Input: part model. Units: mm. Frame: model coordinates. Face numbers are marked on the shaded views. A direction names the side the tool comes from. Give positions to 0.01 mm unless a question says otherwise; leave off trailing zeros. Loops run counter-clockwise (first coordinate to the right, second up) from the corner with the lowest first, then second, coordinate; pieces in that order, holes last.
from build123d import *

# Parameters (mm, degrees)
SKETCH1_R           = 1.65
BOSS_EXTRUDE1_DEPTH = 16
SKETCH2_R           = 2.55
BOSS_EXTRUDE2_DEPTH = 1.5
FILLET1_R           = 2


with BuildPart() as part:
    # Sketch1 → Boss-Extrude1 (new body)
    with BuildSketch(Plane(origin=(76, 0, 0), x_dir=(0, 0, -1), z_dir=(1, 0, 0))):
        Polygon((-39.367141304, -29.396728555), (-62.367141304, -29.396728555), (-62.367141304, -3.396728555), (-56.367141304, -3.396728555), (-56.367141304, -19.796728555), (-39.367141304, -19.796728555), align=None)
        with Locations(Location((-59.367141305, -24.59672823, 0), (0, 0, 90))):
            Circle(SKETCH1_R, mode=Mode.SUBTRACT)
        with Locations(Location((-59.367141305, -6.59672823, 0), (0, 0, 90))):
            Circle(SKETCH1_R, mode=Mode.SUBTRACT)
    extrude(amount=-BOSS_EXTRUDE1_DEPTH)

    # Sketch2 → Boss-Extrude2 (add)
    with BuildSketch(Plane(origin=(0, -19.796728555, 0), x_dir=(1, 0, 0), z_dir=(0, 1, 0))):
        with Locations(Location((64, -51.367141304, 0), (0, 0, 270))):
            Circle(SKETCH2_R)
        with Locations(Location((64, -43.367141304, 0), (0, 0, 270))):
            Circle(SKETCH2_R)
        with Locations(Location((72, -43.367141304, 0), (0, 0, 270))):
            Circle(SKETCH2_R)
        with Locations(Location((72, -51.367141304, 0), (0, 0, 270))):
            Circle(SKETCH2_R)
    extrude(amount=BOSS_EXTRUDE2_DEPTH)

    # Fillet1
    fillet1_edges = [part.edges().sort_by_distance(p)[0] for p in [
        (68, -29.396728555, 62.367141304),
        (68, -3.396728555, 62.367141304),
        (68, -3.396728555, 56.367141304),
    ]]
    fillet(fillet1_edges, radius=FILLET1_R)


solid = part.part
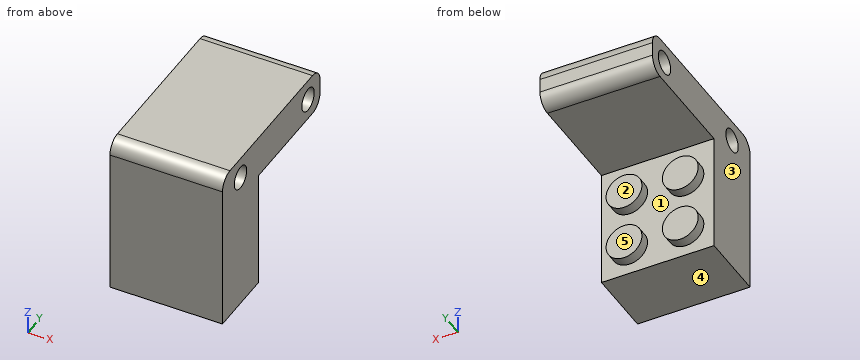
(1) Cut plane A-A (y = -23.75). Return the cut outline in (x, z).
Values follow:
outline: (60, 39.37) - (76, 39.37) - (76, 57.95) - (60, 57.95) - close; (60, 60.78) - (76, 60.78) - (76, 62.37) - (60, 62.37) - close
(2) Ray query, probe 1 along Y at (x, z) = (71.75, 49.75); probe 2 along Z at (x, y) = (66.25, -19.5); probe 3 along Y at (x, z) = (63, 47.75). Return the intervals inside material, ascending.
Values follow:
probe 1: y = -29.4 to -18.3
probe 2: z = 42.17 to 44.57, 50.17 to 52.57, 56.37 to 62.37
probe 3: y = -29.4 to -19.8
(3) Cut plane B-B (x = 72). Return the cut outline in (y, z).
Values follow:
outline: (-29.4, 39.37) - (-19.8, 39.37) - (-19.8, 40.82) - (-18.3, 40.82) - (-18.3, 45.92) - (-19.8, 45.92) - (-19.8, 48.82) - (-18.3, 48.82) - (-18.3, 53.92) - (-19.8, 53.92) - (-19.8, 56.37) - (-5.4, 56.37) arc R2 ccw to (-3.4, 58.37) - (-3.4, 60.37) arc R2 ccw to (-5.4, 62.37) - (-27.4, 62.37) arc R2 ccw to (-29.4, 60.37) - close; hole circle Ø3.3 at (-24.6, 59.37); hole circle Ø3.3 at (-6.6, 59.37)
(4) Cut plane C-C (z = 43.25). Return the cut outline in (x, y).
Values follow:
outline: (60, -29.4) - (76, -29.4) - (76, -19.8) - (74.55, -19.8) - (74.55, -18.3) - (69.45, -18.3) - (69.45, -19.8) - (66.55, -19.8) - (66.55, -18.3) - (61.45, -18.3) - (61.45, -19.8) - (60, -19.8) - close
(5) Reachability of the marked faces 4 and 5 from +Z, -Z, +X, -X, +Y, -Y: full face, straight path, thin tool, end or side. Return the list, or none.
Values follow:
face 4: -Z, +X, -X, +Y, -Y
face 5: -Z, +X, -X, +Y
(6) Cut plane D-D (y = -11.5). Return the cut outline in (x, z).
Values follow:
outline: (60, 56.37) - (76, 56.37) - (76, 62.37) - (60, 62.37) - close
(7) Pin query (flat end, axial travel): pin 1 Ø4 at (x, z) = (73, 42) entering from +Y; pin 2 Ø1 at (x, y) = (65.5, -10.5) entering from -Z; pin 3 Ø1.5 at (x, z) = (73.5, 57) entering from +Y. Return the tip coordinate at first contact, or that it passes through.
Values follow:
pin 1: stops at y = -18.3
pin 2: stops at z = 56.37
pin 3: stops at y = -3.49
(8) Mould query, pull axis X, two halves, no side actions, for the marked faces 1, 2 and 3. Classes: +X half, -X half, draft (parallel to the pull), parting line (faces both ways), or undercut.
Values follow:
face 1: undercut
face 2: draft
face 3: -X half
